Input: part model. Units: mm. Frame: model coordinates. Coordinates: 2 decimals unless noted, no trailing zeros. Loops run counter-clockwise (first coordinate to the right, second up) from the corner with the lowest first, then second, coordinate; pieces in that order, holes last. Notation, with made-up numbers: (16, 29) -> (44, 29) arc R33 ccw to (44, 61) -> close; hole circle Ø4 at (-20.75, 6.25). An arc over 180 degrees is marked (long way). Answer as a JSON object with one key per item and string values.
from build123d import *

# Parameters (mm, degrees)
SKETCH1_W                      = 60
SKETCH1_H                      = 2600
BASE_FLANGE1_DEPTH             = 2
EDGE_FLANGE1_STRIP_W           = 13
EDGE_FLANGE1_STRIP_H           = 2
EDGE_FLANGE1_STRIP_CUT_DEPTH   = 2600
EDGE_FLANGE1_STRIP_2_W         = 13
EDGE_FLANGE1_STRIP_2_H         = 2
EDGE_FLANGE1_STRIP_CUT_2_DEPTH = 2600
EDGE_FLANGE1_DEPTH             = 2600
EDGE_FLANGE1_BEND_DEPTH        = 2600
EDGE_FLANGE2_STRIP_W           = 13
EDGE_FLANGE2_STRIP_H           = 2
EDGE_FLANGE2_STRIP_CUT_DEPTH   = 2600
EDGE_FLANGE2_STRIP_2_W         = 13
EDGE_FLANGE2_STRIP_2_H         = 2
EDGE_FLANGE2_STRIP_CUT_2_DEPTH = 2600
EDGE_FLANGE2_DEPTH             = 2600
EDGE_FLANGE2_BEND_DEPTH        = 2600
SKETCH18_R                     = 5.5
CUT_EXTRUDE1_DEPTH             = 1302.998463901


# Sheet-metal steps are written as plain solids
with BuildPart() as part:
    # Sketch1 → Base-Flange1 (new body)
    with BuildSketch(Plane.XY):
        Rectangle(SKETCH1_W, SKETCH1_H)
    extrude(amount=-BASE_FLANGE1_DEPTH)

    # Edge-Flange1 strip (across the edge) → Edge-Flange1 strip cut (cut)
    with BuildSketch(Plane(origin=(30, 1300, -2), x_dir=(-1, 0, 0), z_dir=(0, -1, 0))):
        with Locations((-2, -1)):
            Rectangle(EDGE_FLANGE1_STRIP_W, EDGE_FLANGE1_STRIP_H)
    extrude(amount=EDGE_FLANGE1_STRIP_CUT_DEPTH, mode=Mode.SUBTRACT)

    # Edge-Flange1 strip 2 (across the edge) → Edge-Flange1 strip cut 2 (cut)
    with BuildSketch(Plane(origin=(-30, -1300, -2), x_dir=(1, 0, 0), z_dir=(0, 1, 0))):
        with Locations((-2, -1)):
            Rectangle(EDGE_FLANGE1_STRIP_2_W, EDGE_FLANGE1_STRIP_2_H)
    extrude(amount=EDGE_FLANGE1_STRIP_CUT_2_DEPTH, mode=Mode.SUBTRACT)

    # Edge-Flange1 section (across the edge) → Edge-Flange1 (add)
    with BuildSketch(Plane(origin=(30, 1300, -2), x_dir=(-1, 0, 0), z_dir=(0, -1, 0))):
        with BuildLine():
            Line((0, 2.5), (0, 38))
            Line((0, 38), (2, 38))
            Line((2, 38), (2, 2.5))
            ThreePointArc((2, 2.5), (2.732233047, 0.732233047), (4.5, 0))
            Line((4.5, 0), (4.5, -2))
            ThreePointArc((4.5, -2), (1.318019485, -0.681980515), (0, 2.5))
        make_face()
    extrude(amount=EDGE_FLANGE1_DEPTH)

    # Edge-Flange1 section 2 (across the edge) → Edge-Flange1 bend (add)
    with BuildSketch(Plane(origin=(-30, -1300, -2), x_dir=(1, 0, 0), z_dir=(0, 1, 0))):
        with BuildLine():
            Line((0, 2.5), (0, 38))
            Line((0, 38), (2, 38))
            Line((2, 38), (2, 2.5))
            ThreePointArc((2, 2.5), (2.732233047, 0.732233047), (4.5, 0))
            Line((4.5, 0), (4.5, -2))
            ThreePointArc((4.5, -2), (1.318019485, -0.681980515), (0, 2.5))
        make_face()
    extrude(amount=EDGE_FLANGE1_BEND_DEPTH)

    # Edge-Flange2 strip (across the edge) → Edge-Flange2 strip cut (cut)
    with BuildSketch(Plane(origin=(28, 1300, -40), x_dir=(0, 0, 1), z_dir=(0, -1, 0))):
        with Locations((-2, -1)):
            Rectangle(EDGE_FLANGE2_STRIP_W, EDGE_FLANGE2_STRIP_H)
    extrude(amount=EDGE_FLANGE2_STRIP_CUT_DEPTH, mode=Mode.SUBTRACT)

    # Edge-Flange2 strip 2 (across the edge) → Edge-Flange2 strip cut 2 (cut)
    with BuildSketch(Plane(origin=(-28, -1300, -40), x_dir=(0, 0, 1), z_dir=(0, 1, 0))):
        with Locations((-2, -1)):
            Rectangle(EDGE_FLANGE2_STRIP_2_W, EDGE_FLANGE2_STRIP_2_H)
    extrude(amount=EDGE_FLANGE2_STRIP_CUT_2_DEPTH, mode=Mode.SUBTRACT)

    # Edge-Flange2 section (across the edge) → Edge-Flange2 (add)
    with BuildSketch(Plane(origin=(28, 1300, -40), x_dir=(0, 0, 1), z_dir=(0, -1, 0))):
        with BuildLine():
            Line((0, 2.5), (0, 11))
            Line((0, 11), (2, 11))
            Line((2, 11), (2, 2.5))
            ThreePointArc((2, 2.5), (2.732233047, 0.732233047), (4.5, 0))
            Line((4.5, 0), (4.5, -2))
            ThreePointArc((4.5, -2), (1.318019485, -0.681980515), (0, 2.5))
        make_face()
    extrude(amount=EDGE_FLANGE2_DEPTH)

    # Edge-Flange2 section 2 (across the edge) → Edge-Flange2 bend (add)
    with BuildSketch(Plane(origin=(-28, -1300, -40), x_dir=(0, 0, 1), z_dir=(0, 1, 0))):
        with BuildLine():
            Line((0, 2.5), (0, 11))
            Line((0, 11), (2, 11))
            Line((2, 11), (2, 2.5))
            ThreePointArc((2, 2.5), (2.732233047, 0.732233047), (4.5, 0))
            Line((4.5, 0), (4.5, -2))
            ThreePointArc((4.5, -2), (1.318019485, -0.681980515), (0, 2.5))
        make_face()
    extrude(amount=EDGE_FLANGE2_BEND_DEPTH)

    # Sketch18 → Cut-Extrude1 (cut, symmetric)
    with BuildSketch(Plane(origin=(30, 0, 0), x_dir=(0, 0, -1), z_dir=(1, 0, 0))):
        with Locations(Location((20, 1255, 0), (0, 0, 180))):
            Circle(SKETCH18_R)
        with Locations(Location((20, 1285, 0), (0, 0, 180))):
            Circle(SKETCH18_R)
    cut_extrude1 = extrude(amount=CUT_EXTRUDE1_DEPTH, both=True, mode=Mode.SUBTRACT)

    # Mirror1: Cut-Extrude1 across plane
    add(cut_extrude1.mirror(Plane.ZX), mode=Mode.SUBTRACT)


solid = part.part
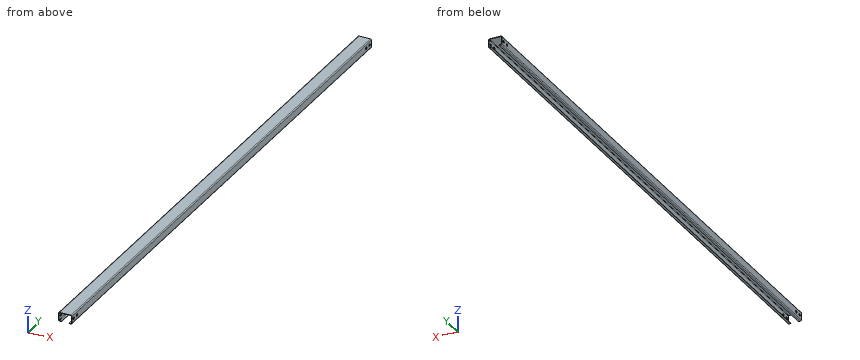
1. Section query A-A (y = -10). Return loops of the section in (x, z).
Reply:
{"outline": "(-30, -35.5) arc R4.5 ccw to (-25.5, -40) -> (-17, -40) -> (-17, -38) -> (-25.5, -38) arc R2.5 cw to (-28, -35.5) -> (-28, -4.5) arc R2.5 cw to (-25.5, -2) -> (25.5, -2) arc R2.5 cw to (28, -4.5) -> (28, -35.5) arc R2.5 cw to (25.5, -38) -> (17, -38) -> (17, -40) -> (25.5, -40) arc R4.5 ccw to (30, -35.5) -> (30, -4.5) arc R4.5 ccw to (25.5, 0) -> (-25.5, 0) arc R4.5 ccw to (-30, -4.5) -> close"}
2. Line query: line 1 along Y through (x, z) = (-29.6, -20); line 2 along X through (y, z) = (-189.5, -4.5); line 3 along Z through (x, y) = (21.5, -1122). Output: solid intervals per line, ascending.
Reply:
{"line 1": "y = -1300 to -1290.5, -1279.5 to -1260.5, -1249.5 to 1249.5, 1260.5 to 1279.5, 1290.5 to 1300", "line 2": "x = -30 to -28, 28 to 30", "line 3": "z = -40 to -38, -2 to 0"}
3. Pin query (flat end, axial travel): P1, Ø10, axis at x = 7.5, y = -263.5, coming from the +Z side; P2, Ø1.6, axis at y = 164.5, z = -39, coming from the -X side; P3, Ø10, axis at x = -5.5, y = 304, coming from the -Z side; P4, Ø1.6, axis at y = 619.5, z = -39, coming from the +X side. Return the tip coordinate at first contact, or that it passes through.
Reply:
{"P1": "stops at z = 0", "P2": "stops at x = -29.1", "P3": "stops at z = -2", "P4": "stops at x = 29.1"}
4. Section query B-B (x = 4). Return loops of the section in (y, z), plus the area to 3 significant figures.
Reply:
{"outline": "(-1300, -2) -> (1300, -2) -> (1300, 0) -> (-1300, 0) -> close", "area": "5,200 mm2"}
